Model file for the job. Use its own axes, mm. Round coordinates to 2 decimals unless told otherwise and drop trailing zeros. Loops run counter-clockwise (first coordinate to the right, second up) from the corner with the lowest first, then second, coordinate; pieces in that order, holes last. Notation, with made-up numbers: M 27,67.5 L 70,67.5 A26 ccw 70,96.5 Z; hole C 42,88 d11. An arc over 180 degrees is marked long. Answer in a Markdown table with one row per item.
from build123d import *

# Parameters (mm, degrees)
SKETCH_1_W           = 117
SKETCH_1_H           = 120
EXTRUDE_1_DEPTH      = 4
SKETCH_4_W           = 91
SKETCH_4_H           = 23
CUT_EXTRUDE_3_DEPTH  = 10
CUT_EXTRUDE_4_DEPTH  = 10
SKETCH_6_R           = 1.525
CUT_EXTRUDE_5_DEPTH  = 4
SKETCH_8_R           = 2.525
CUT_EXTRUDE_7_DEPTH  = 40
FILLET_1_R           = 2
CUT_EXTRUDE_10_DEPTH = 4
EXTRUDE_4_DEPTH      = 4
FILLET_4_R           = 2
SKETCH_18_R          = 3
EXTRUDE_6_DEPTH      = 4
SKETCH_19_R          = 1.525
CUT_EXTRUDE_12_DEPTH = 4
EXTRUDE_START        = -4
SKETCH_20_R          = 3
SKETCH_20_R_2        = 1.525
EXTRUDE_7_DEPTH      = 4
FILLET_6_R           = 2
SKETCH_21_R          = 2.025
CUT_EXTRUDE_13_DEPTH = 10


with BuildPart() as part:
    # 草图1 → 凸台-拉伸1 (new body)
    with BuildSketch(Plane.XY):
        Rectangle(SKETCH_1_W, SKETCH_1_H)
    extrude(amount=EXTRUDE_1_DEPTH)

    # 草图4 → 切除-拉伸3 (cut)
    with BuildSketch(Plane(origin=(0, 0, 0), x_dir=(-1, 0, 0), z_dir=(0, 0, -1))):
        with Locations((0, -35.5)):
            Rectangle(SKETCH_4_W, SKETCH_4_H)
    extrude(amount=-CUT_EXTRUDE_3_DEPTH, mode=Mode.SUBTRACT)

    # 草图5 → 切除-拉伸4 (cut)
    with BuildSketch(Plane.XY.offset(4)):
        Polygon((-52.5, 60), (-40.5, 30), (40.5, 30), (52.5, 60), align=None)
    extrude(amount=-CUT_EXTRUDE_4_DEPTH, mode=Mode.SUBTRACT)

    # 草图6 → 切除-拉伸5 (cut)
    with BuildSketch(Plane(origin=(0, 0, 0), x_dir=(-1, 0, 0), z_dir=(0, 0, -1))):
        with Locations((-55.5, 21)):
            Circle(SKETCH_6_R)
        with Locations((-55.5, 1)):
            Circle(SKETCH_6_R)
    cut_extrude_5 = extrude(amount=-CUT_EXTRUDE_5_DEPTH, mode=Mode.SUBTRACT)

    # 镜向1: 切除-拉伸5 across plane
    add(cut_extrude_5.mirror(Plane(origin=(0, 0, 0), x_dir=(0, 0, 1), z_dir=(1, 0, 0))), mode=Mode.SUBTRACT)

    # 草图8 → 切除-拉伸7 (cut)
    with BuildSketch(Plane(origin=(0, 0, 0), x_dir=(-1, 0, 0), z_dir=(0, 0, -1))):
        with Locations((30, -54)):
            Circle(SKETCH_8_R)
        with Locations((-30, -54)):
            Circle(SKETCH_8_R)
    extrude(amount=-CUT_EXTRUDE_7_DEPTH, mode=Mode.SUBTRACT)

    # 圆角1
    fillet_1_edges = [part.edges().sort_by_distance(p)[0] for p in [
        (-45.5, -47, 2),
        (45.5, -47, 2),
        (45.5, -24, 2),
        (-45.5, -24, 2),
        (-52.5, 60, 2),
        (52.5, 60, 2),
        (40.5, 30, 2),
        (-40.5, 30, 2),
        (58.5, -60, 2),
        (-58.5, -60, 2),
        (-58.5, 60, 2),
        (58.5, 60, 2),
    ]]
    fillet(fillet_1_edges, radius=FILLET_1_R)

    # 草图12 → 切除-拉伸10 (cut)
    with BuildSketch(Plane(origin=(0, 0, 0), x_dir=(-1, 0, 0), z_dir=(0, 0, -1))):
        Polygon((49.5, 21.428623254), (3.182078723, -16), (49.5, -16), align=None)
        Polygon((2, 24), (2, -11.812461638), (46.317921277, 24), align=None)
        Polygon((-46.317921277, 24), (-2, -11.812461638), (-2, 24), align=None)
        Polygon((-49.5, -16), (-3.182078723, -16), (-49.5, 21.428623254), align=None)
    extrude(amount=-CUT_EXTRUDE_10_DEPTH, mode=Mode.SUBTRACT)

    # 草图15 → 凸台-拉伸4 (add)
    with BuildSketch(Plane.XY.offset(4)):
        Polygon((-3.288271492, 25.529822396), (-50.788271492, -14.470177604), (-48.211728508, -17.529822396), (-0.711728508, 22.470177604), align=None)
        Polygon((0.711728508, 22.470177604), (48.211728508, -17.529822396), (50.788271492, -14.470177604), (3.288271492, 25.529822396), align=None)
    extrude(amount=-EXTRUDE_4_DEPTH)

    # 圆角4
    fillet_4_edges = [part.edges().sort_by_distance(p)[0] for p in [
        (-2, -11.812461638, 2),
        (-46.317921277, 24, 2),
        (46.317921277, 24, 2),
        (2, -11.812461638, 2),
        (3.182078723, -16, 2),
        (49.5, 21.428623254, 2),
        (-3.182078723, -16, 2),
        (-49.5, 21.428623254, 2),
        (-22.117597413, 4.444182736, 2),
        (-25.286552291, 7.004954355, 2),
        (-28.403021143, 4.380559532, 2),
        (-5.104935587, 24, 2),
        (-25.234066266, 1.819787913, 2),
        (-2, 21.3853174, 2),
        (-49.5, -13.3853174, 2),
        (-46.395064413, -16, 2),
        (25.286552291, 7.004954355, 2),
        (22.117597413, 4.444182736, 2),
        (25.234066266, 1.819787913, 2),
        (2, 21.3853174, 2),
        (5.104935587, 24, 2),
        (46.395064413, -16, 2),
        (49.5, -13.3853174, 2),
        (28.403021143, 4.380559532, 2),
    ]]
    fillet(fillet_4_edges, radius=FILLET_4_R)

    # 草图18 → 凸台-拉伸6 (add)
    with BuildSketch(Plane(origin=(0, 0, 0), x_dir=(-1, 0, 0), z_dir=(0, 0, -1))):
        with Locations((20, 4)):
            Circle(SKETCH_18_R)
    extrude(amount=-EXTRUDE_6_DEPTH)

    # 草图19 → 切除-拉伸12 (cut)
    with BuildSketch(Plane.XY.offset(4)):
        with Locations((0, 4)):
            Circle(SKETCH_19_R)
        with Locations((-20, 4)):
            Circle(SKETCH_19_R)
    extrude(amount=-CUT_EXTRUDE_12_DEPTH, mode=Mode.SUBTRACT)

    # 草图20 → 凸台-拉伸7 (add)
    with BuildSketch(Plane(origin=(0, 0, 0), x_dir=(-1, 0, 0), z_dir=(0, 0, -1)).offset(EXTRUDE_START)):
        with Locations((0, 4)):
            Circle(SKETCH_20_R)
        with Locations(Location((0, 4, 0), (0, 0, 180))):
            Circle(SKETCH_20_R_2, mode=Mode.SUBTRACT)
    extrude(amount=EXTRUDE_7_DEPTH)

    # 圆角6
    fillet_6_edges = [part.edges().sort_by_distance(p)[0] for p in [
        (-19.208718836, 6.893764697, 2),
        (-18.415492277, 1.452582626, 2),
        (-2, 6.236067977, 2),
        (-2, 1.763932023, 2),
        (2, 1.763932023, 2),
        (2, 6.236067977, 2),
    ]]
    fillet(fillet_6_edges, radius=FILLET_6_R)

    # 草图21 → 切除-拉伸13 (cut)
    with BuildSketch(Plane.XY.offset(4)):
        with Locations((-15, -54)):
            Circle(SKETCH_21_R)
        with Locations((15, -54)):
            Circle(SKETCH_21_R)
    extrude(amount=-CUT_EXTRUDE_13_DEPTH, mode=Mode.SUBTRACT)


solid = part.part
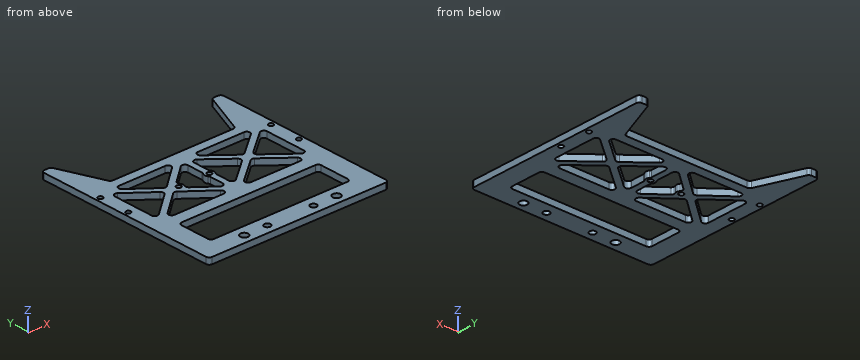
1. Wall check: probe 1 along Y at (x, z) = (-55.5, 2.95) (3 decimals); probe 2 along Y at (x, z) = (7, 2.2); probe 3 along X at (y, z) = (-12.5, 3). Give the ranges that are in metal, low to high.
Verdict:
| item | result |
|---|---|
| probe 1 | y = -60 to -0.525, 2.525 to 19.475, 22.525 to 60 |
| probe 2 | y = -60 to -47, -24 to -14.79, -13.21 to -7.77, 17.17 to 30 |
| probe 3 | x = -58.5 to -42.24, -7.52 to 7.52, 42.24 to 58.5 |
2. Saw through at B-B (y = 47.5). Write the cut outline in (x, z), and give its area (3 significant figures).
Verdict:
| item | result |
|---|---|
| outline | M -58.5,0 L -47.5,0 L -47.5,4 L -58.5,4 Z; M 47.5,0 L 58.5,0 L 58.5,4 L 47.5,4 Z |
| area | 88.0 mm² |
3. Saw through at C-C (x = 15). Write the cut outline in (y, z) (3 decimals), and give its area (3 significant figures).
Verdict:
| item | result |
|---|---|
| outline | M -60,0 L -56.025,0 L -56.025,4 L -60,4 Z; M -51.975,0 L -47,0 L -47,4 L -51.975,4 Z; M -24,0 L -16,0 L -16,4 L -24,4 Z; M -6.45,0 L -1.307,0 L -1.307,4 L -6.45,4 Z; M 10.438,0 L 15.667,0 L 15.667,4 L 10.438,4 Z; M 24,0 L 30,0 L 30,4 L 24,4 Z |
| area | 133 mm² |
4. Saw through at A-A (y = -54). Write the cut outline in (x, z) (3 decimals).
Verdict:
| item | result |
|---|---|
| outline | M -58.5,0 L -32.525,0 L -32.525,4 L -58.5,4 Z; M -27.475,0 L -17.025,0 L -17.025,4 L -27.475,4 Z; M -12.975,0 L 12.975,0 L 12.975,4 L -12.975,4 Z; M 17.025,0 L 27.475,0 L 27.475,4 L 17.025,4 Z; M 32.525,0 L 58.5,0 L 58.5,4 L 32.525,4 Z |
5. Saw through at D-D (x = -20). Write the cut outline in (y, z) (3 decimals), and give its area (3 significant figures).
Verdict:
| item | result |
|---|---|
| outline | M -60,0 L -47,0 L -47,4 L -60,4 Z; M -24,0 L -16,0 L -16,4 L -24,4 Z; M -2.41,0 L 2.475,0 L 2.475,4 L -2.41,4 Z; M 5.525,0 L 11.457,0 L 11.457,4 L 5.525,4 Z; M 24,0 L 30,0 L 30,4 L 24,4 Z |
| area | 151 mm² |
6. Pin check, flat tips, straight feed: pin 1 (2.5 mm diameter, centred on x = -20, y = 4, fed in from +Z); pin 2 (2 mm diameter, centred on x = 20.5, z = 2.5, fed in from +Y). Stop position of each tip, or through.
Verdict:
| item | result |
|---|---|
| pin 1 | passes through |
| pin 2 | stops at y = 30 |
